Autodesk Inventor part; units mm, degrees
ref_plane "YZ Plane" through (0, 0, 0) normal (1, 0, 0) x (0, 1, 0)
ref_plane "XZ Plane" through (0, 0, 0) normal (0, 1, 0) x (-1, 0, 0)
ref_plane "XY Plane" through (0, 0, 0) normal (0, 0, 1) x (1, 0, 0)
sketch "Sketch1" plane through (0, 0, 0) normal (0, 0, 1) x (1, 0, 0)
  point P0 (0, 0)
sketch "Sketch2" plane through (0, 0, 0) normal (0, 0, 1) x (1, 0, 0)
  circle A0 centre (0, 0) radius 210
  dimension "d0" = 420
extrude "Extrusion1" add sketch "Sketch2" along normal blind 20
sketch "Sketch3" plane through (0, 0, 20) normal (0, 0, 1) x (1, 0, 0)
  circle A0 centre (0, 0) radius 25
  circle A1 centre (0, 0) radius 15.875
  dimension "d6" = 50
  dimension "d7" = 31.75
extrude "Extrusion2" add sketch "Sketch3" along normal blind 30
extrude "Extrusion3" cut sketch "Sketch3" against normal blind 20 contours A1
sketch "Sketch4" plane through (0, 0, 20) normal (0, 0, 1) x (1, 0, 0)
  circle A0 centre (0, 0) radius 15.875
  circle A1 centre (0, 0) radius 180
  circle A2 centre (0, 195) radius 10
  dimension "d12" = 360
  dimension "d13" = 20
  dimension "d23" = 195
extrude "Extrusion4" cut sketch "Sketch4" against normal blind 20 contours A2
sketch "Sketch5" plane through (0, 0, 50) normal (0, 0, 1) x (1, 0, 0)
  line L0 (-5, 13.375) -> (5, 13.375)
  line L1 (5, 13.375) -> (5, 18.375)
  line L2 (5, 18.375) -> (-5, 18.375)
  line L3 (-5, 18.375) -> (-5, 13.375)
  circle A0 centre (0, 0) radius 15.875
  line L4 (-5, 13.375) -> (5, 18.375) construction
  line L5 (5, 13.375) -> (-5, 18.375) construction
  point P0 (0, 15.875)
  point P1 (-5, 15.067)
  point P2 (5, 15.067)
  dimension "d19" = 10
  dimension "d20" = 5
extrude "Extrusion5" add sketch "Sketch5" against normal blind 30 contours L3 A0 L1 L0 | L3 L2 L1 A0 picked at (-0.5641, 14.1782)
pattern_circular "Circular Pattern1" count 4 over 360 about axis through (0, 0, 0) along (0, 0, 1) of "Extrusion4"
properties part number "Rotary Motor Coupling"
Geometry check sheet. Reference: the model listing, model coordinates, mm. A direction names the side the tool comes from. Coordinates: 2 decimals unless noted, no trailing zeros. Order: outer loops, then holes, each group sorted by start corner. A loop starts at its lowest first (then second) coordinate and runs counter-clockwise, first axis right, second up. Notation, with made-up numbers: (57.5, -23.5) - (71.5, -23.5) arc R8 ccw to (71.5, -11.5) - close; hole circle Ø2 at (8, 69). An arc over 180 degrees is marked (long way). Answer as a JSON object with one key per item and string values. Group by question number.
Item 1: Sectioned sample at A-A, the plane y = 0. Record the cut outline in (x, z) (3 decimals).
Item 2: Sectioned sample at C-C, the plane x = 195. Record the cut outline in (y, z).
Item 3: Depth check by flat-ended pin: pin 1 Ø10 at (y, z) = (110.5, 24) entering from -X; pin 2 Ø1.9 at (y, z) = (14, 35) entering from +X; pin 3 Ø1 at (x, y) = (94.5, 147) entering from +Z; pin 4 Ø23 at (x, y) = (195, 0) entering from -Z. Enter the tip coordinate at first touch or a pass-through.
Item 4: Draft check along X on faces 4 (the face through (200.3, -63.08, 9.86)), 5 (the face through (-3, -44, 20)), 6 (the face through (2.17, -185.24, 10.14)). Enter one of: +X half, -X half, draft (parallel to the pull), parting line (faces both ways), or undercut.
Item 5: Tool access check on faces 1 (the face through (23.846, -7.509, 34.79)), 2 (the face through (-0.3, -16.3, 50)), 3 (the face through (0, 13.375, 35)). Record the directions out of +Z, -Z, +X, -X, +Y, -Y that give a thin tool (end or side, any length) a straight path to the whole face; none if there is none.
Item 6: Scan lines: probe 1 along Y at (x, z) = (0, 15.75) (3 decimals); probe 2 along Z at (x, y) = (102, 17); probe 3 along X at (y, z) = (12.5, 4). Record each from-to range of solid material in increasing order.
Item 7: Sectioned sample at B-B, the plane x = 0. Record the cut outline in (y, z) (3 decimals).
Resolved:
{
 "1": {"outline": "(-210, 0) - (-205, 0) - (-205, 20) - (-210, 20) - close; (-185, 0) - (-15.875, 0) - (-15.875, 50) - (-25, 50) - (-25, 20) - (-185, 20) - close; (15.875, 0) - (185, 0) - (185, 20) - (25, 20) - (25, 50) - (15.875, 50) - close; (205, 0) - (210, 0) - (210, 20) - (205, 20) - close"},
 "2": {"outline": "(-77.94, 0) - (-10, 0) - (-10, 20) - (-77.94, 20) - close; (10, 0) - (77.94, 0) - (77.94, 20) - (10, 20) - close"},
 "3": {"pin 1": "x = -180.4", "pin 2": "x = 21.32", "pin 3": "z = 20", "pin 4": "z = 0"},
 "4": {"face 4": "parting line", "face 5": "draft", "face 6": "undercut"},
 "5": {"face 1": "+Z", "face 2": "+Z, +X, -X, +Y, -Y", "face 3": "+Z, -Z"},
 "6": {"probe 1": "-210 to -205, -185 to -15.875, 15.875 to 185, 205 to 210", "probe 2": "0 to 20", "probe 3": "-209.63 to -9.79, 9.79 to 209.63"},
 "7": {"outline": "(-210, 0) - (-205, 0) - (-205, 20) - (-210, 20) - close; (-185, 0) - (-15.875, 0) - (-15.875, 50) - (-25, 50) - (-25, 20) - (-185, 20) - close; (13.375, 20) - (15.875, 20) - (15.875, 0) - (185, 0) - (185, 20) - (25, 20) - (25, 50) - (13.375, 50) - close; (205, 0) - (210, 0) - (210, 20) - (205, 20) - close"}
}
